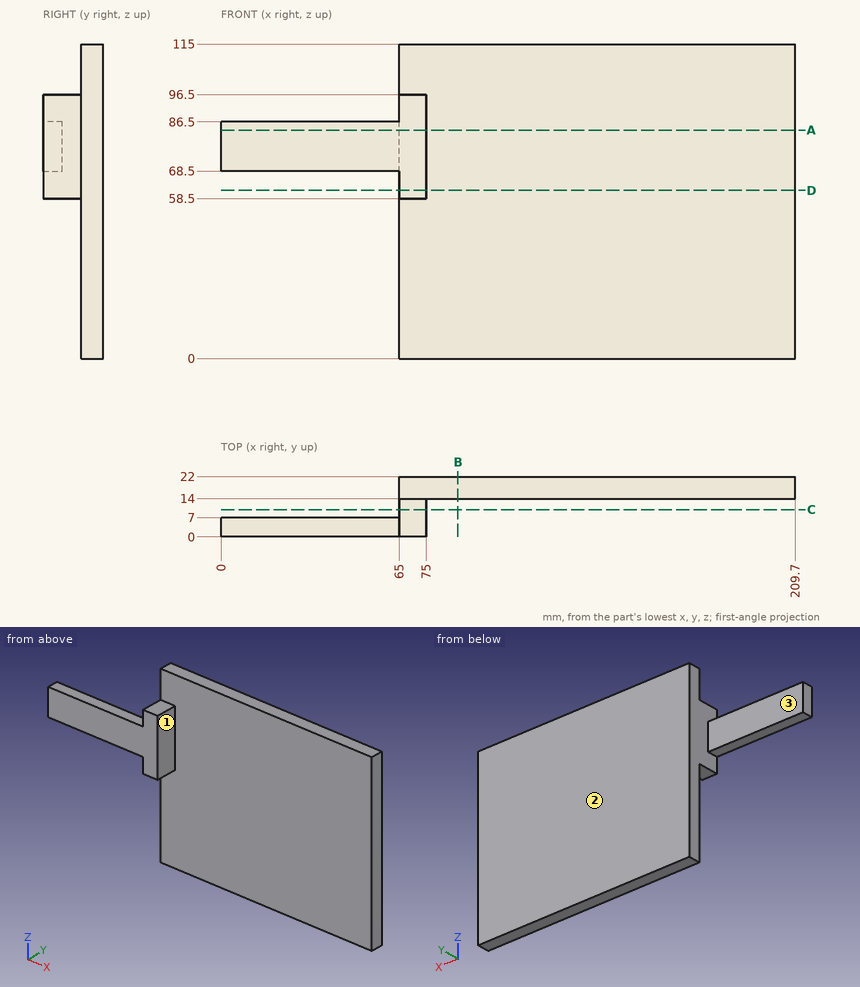
Input: dimensioned drawing with shaded views. Units: mm. Origin: part minimum x, y, z. A direction names the side the tool comes from. Round coordinates to 2 decimals unless told otherwise and drop trailing zeros. Loops run counter-clockwise (first coordinate to the right, second up) from the corner with the lowest first, then second, coordinate; pieces in that order, holes last. Notation, with made-up numbers: M -12.75,-38 L 37.25,-38 A16 cw 37.25,-16 Z; hole C 13.5,10 d8. An arc over 180 degrees is marked long. One line per question, with ' | ' between items.
(1) Material intervals for line 1 along X through (y, z) = (6.5, 96); line 2 along Y through (x, z) = (198.5, 11.5); line 3 along Z through (x, y) = (52.5, 1.25), sorted ascending. Write a range as from..to.
Check result:
line 1: x = 65..75 | line 2: y = 14..22 | line 3: z = 68.5..86.5
(2) Access query for the marked faces 1, 2 and 3. Directions: +Z, -Z, +X, -X, +Y, -Y. A direction counts if a zero-diameter tool reaches every point of the face in a straight line with its end or side. Return the directions, or none.
Check result:
face 1: +Z, -Z, +X, -Y | face 2: +Z, -Z, +X, -X, +Y | face 3: +Z, -Z, -X, +Y
(3) Cut plane D-D on z = 61.5. Return the cut outline in (x, y), plus the area to 3 significant figures.
Check result:
outline: M 65,0 L 75,0 L 75,14 L 209.7,14 L 209.7,22 L 65,22 Z | area: 1,300 mm2
(4) Cut plane B-B on x = 86.5. Return the cut outline in (y, z), plus the area to 3 significant figures.
Check result:
outline: M 14,0 L 22,0 L 22,115 L 14,115 Z | area: 920 mm2
(5) Cut plane A-A on z = 83.5. Return the cut outline in (x, y), plus the area to 3 significant figures.
Check result:
outline: M 0,0 L 75,0 L 75,14 L 209.7,14 L 209.7,22 L 65,22 L 65,7 L 0,7 Z | area: 1,750 mm2
(6) Contact query for flat-ended pins moving along their axis: P1, Ø8, axis at x = 70, y = 4.5, coming from the -Z side; P2, Ø2, axis at x = 28, y = 2, coming from the +Z side; P3, Ø5, axis at y = 14, z = 40.5, coming from the -X side; P4, Ø6, axis at x = 154.5, y = 10.5, coming from the +Z side. Output: stop coordinate, or through.
Check result:
P1: stops at z = 58.5 | P2: stops at z = 86.5 | P3: stops at x = 65 | P4: passes through
(7) Cut plane C-C on y = 10. Return the cut outline in (x, z), plus the area to 3 significant figures.
Check result:
outline: M 65,58.5 L 75,58.5 L 75,96.5 L 65,96.5 Z | area: 380 mm2
